Can you work these out from the model? Positions are in its coordinate system, mm. A direction names the side the tool comes from. Give positions to 0.01 mm unless a question says otherwise; leave off trailing zeros. Order: outer loops, then holes, each group sorted by start corner. A loop starts at its lowest first (then second) coordinate and runs counter-clockwise, first axis right, second up. Notation, with made-up numbers: M -39.5,50.25 L -24.5,50.25 A20 cw -24.5,80.25 Z; hole C 46.5,16 d1. An arc over 180 degrees is marked long. Use one line per item in the form item = value. Start each with the question number.
1. I need wall thicknesses on L1, parallel to X at y = 34.5, z = 57; L2, parallel to X at y = 75.5, z = 4.5; L3, parallel to Z at x = 164, y = 23. Which ranges of each line are inside material? Lowest first, please.
2. Will these pins go through, and if not, where does the flat tip stop? P1, Ø2, axis at y = 56, z = 12, coming from the +X side; P2, Ø8, axis at x = 34, z = 22.5, coming from the -Y side; P3, Ø1.6, axis at y = 83, z = 2, coming from the +X side; P4, Ø6, axis at x = -20.26, y = 0, coming from the +Z side.
3. I want a section at C-C, the plane z = 12. List the corners of the cut face in (x, y) for me, and give its area (3 significant figures).
4. I want a section at A-A, the plane x = 8.5. List the corners of the cut face in (y, z) for me, and give its area (3 significant figures).
5. For faces 4 (the face through (71.21, 54.46, 37.16)), 5 (the face through (71.14, -21.95, 19.46)), 6 (the face through (0, 82, 3)), 7 (the face through (142.16, 30.54, 65.24)), 8 (the face through (143.2, -15.65, 23.61)), which set-ups out of +Z, -Z, +X, -X, +Y, -Y let a thin tool reach every point of the face, with its end or its side?
6. We'd pull the mould along X, two halves only. Please class faces 1 (the face through (175.739, 24, 3)), 2 (the face through (-2.65, 32.53, 66.63)), 3 (the face through (72, -21, 7)): +X half, -X half, draft (parallel to the pull), parting line (faces both ways), or undercut.
```python
from build123d import *

# Parameters (mm, degrees)
F0_R          = 3.25
F0_W          = 147
F0_H          = 74
F0_W_2        = 5
F0_H_2        = 3
F1_DEPTH      = 7
F4_DEPTH      = 150.739
F4_DEPTH_BACK = 6.261
F5_W          = 147
F5_H          = 67.7437671193
F6_DEPTH      = 156.2
F7_R          = 1
F9_DEPTH      = 15
F10_R         = 1.75
F11_DEPTH     = 15


# Not quite as in the source:
# - a feature names something its author has since deleted; it is built from what else it names


with BuildPart() as f1:
    # F0 (on Top) → F1 (new body)
    with BuildSketch(Plane.XY):
        Polygon((30.7393903136, 82), (-31.2606096864, 82), (-31.2606096864, -32), (175.7393903136, -32), (175.7393903136, 82), (113.7393903136, 82), (108.7393903136, 82), (35.7393903136, 82), align=None)
        with Locations((-20.2606096864, 0)):
            Circle(F0_R, mode=Mode.SUBTRACT)
        with Locations((164.7393903136, 0)):
            Circle(F0_R, mode=Mode.SUBTRACT)
        with Locations((72.2393903136, 30)):
            Rectangle(F0_W, F0_H, mode=Mode.SUBTRACT)
        with Locations((33.2393903136, 83.5)):
            Rectangle(F0_W_2, F0_H_2)
        with Locations((111.2393903136, 83.5)):
            Rectangle(F0_W_2, F0_H_2)
    extrude(amount=F1_DEPTH)

    # F3 (on Right) → F4 (join, two sides)
    with BuildSketch(Plane.YZ) as f4_sk:
        Polygon((-13.2231451571, 7), (81.6844701767, 7), (33.2535275188, 76.1665542214), (-30.4304382476, 31.5745613287), align=None)
    extrude(amount=F4_DEPTH)
    extrude(f4_sk.sketch, amount=-F4_DEPTH_BACK)

    # F5 (on face) → F6 (cut)
    with BuildSketch(Plane(origin=(0, -24.8464988409, 35.4844777942), x_dir=(1, 0, 0), z_dir=(0, -0.5735764364, 0.8191520443))):
        with Locations((72.239, 32.0551522267)):
            Rectangle(F5_W, F5_H)
    extrude(amount=-F6_DEPTH, mode=Mode.SUBTRACT)

    # F7
    f7_edges = [f1.edges().sort_by_distance(p)[0] for p in [
        (111.23939, 85, 7),
        (33.23939, 85, 7),
        (35.73939, 85, 3.5),
        (30.73939, 85, 3.5),
        (108.73939, 85, 3.5),
        (113.73939, 85, 3.5),
    ]]
    fillet(f7_edges, radius=F7_R)

    # F8 (on face) → F9 (join)
    with BuildSketch(Plane(origin=(0, -24.8464988409, 35.4844777942), x_dir=(1, 0, 0), z_dir=(0, -0.5735764364, 0.8191520443))):
        with BuildLine():
            Line((-1.261, 65.9270357864), (3.739, 65.9270357864))
            ThreePointArc((3.739, 65.9270357864), (2.2745339059, 69.4625696923), (-1.261, 70.9270357864))
            Line((-1.261, 70.9270357864), (-6.261, 70.9270357864))
            Line((-6.261, 70.9270357864), (-6.261, 65.9270357864))
            ThreePointArc((-6.261, 65.9270357864), (-4.7965339059, 62.3915018804), (-1.261, 60.9270357864))
            Line((-1.261, 60.9270357864), (-1.261, 65.9270357864))
        make_face()
        with BuildLine():
            ThreePointArc((-1.261, 60.9270357864), (2.2745339059, 62.3915018804), (3.739, 65.9270357864))
            Line((3.739, 65.9270357864), (-1.261, 65.9270357864))
            Line((-1.261, 65.9270357864), (-1.261, 60.9270357864))
        make_face()
        with BuildLine():
            Line((145.739, -1.8167313329), (145.739, 3.1832686671))
            ThreePointArc((145.739, 3.1832686671), (142.2034660941, 1.718802573), (140.739, -1.8167313329))
            Line((140.739, -1.8167313329), (145.739, -1.8167313329))
        make_face()
        with BuildLine():
            ThreePointArc((140.739, 65.9270357864), (142.2034660941, 62.3915018804), (145.739, 60.9270357864))
            Line((145.739, 60.9270357864), (145.739, 65.9270357864))
            Line((145.739, 65.9270357864), (140.739, 65.9270357864))
        make_face()
        with BuildLine():
            Line((150.739, -6.8167313329), (150.739, -1.8167313329))
            ThreePointArc((150.739, -1.8167313329), (149.2745339059, 1.718802573), (145.739, 3.1832686671))
            Line((145.739, 3.1832686671), (145.739, -1.8167313329))
            Line((145.739, -1.8167313329), (140.739, -1.8167313329))
            ThreePointArc((140.739, -1.8167313329), (142.2034660941, -5.3522652388), (145.739, -6.8167313329))
            Line((145.739, -6.8167313329), (150.739, -6.8167313329))
        make_face()
        with BuildLine():
            ThreePointArc((145.739, 60.9270357864), (149.2745339059, 62.3915018804), (150.739, 65.9270357864))
            Line((150.739, 65.9270357864), (150.739, 70.9270357864))
            Line((150.739, 70.9270357864), (145.739, 70.9270357864))
            ThreePointArc((145.739, 70.9270357864), (142.2034660941, 69.4625696923), (140.739, 65.9270357864))
            Line((140.739, 65.9270357864), (145.739, 65.9270357864))
            Line((145.739, 65.9270357864), (145.739, 60.9270357864))
        make_face()
        with BuildLine():
            Line((-1.261, -1.8167313329), (3.739, -1.8167313329))
            ThreePointArc((3.739, -1.8167313329), (2.2745339059, 1.718802573), (-1.261, 3.1832686671))
            Line((-1.261, 3.1832686671), (-1.261, -1.8167313329))
        make_face()
    extrude(amount=-F9_DEPTH)

    # F10 (on face) → F11 (cut)
    with BuildSketch(Plane(origin=(0, -24.8464988409, 35.4844777942), x_dir=(1, 0, 0), z_dir=(0, -0.5735764364, 0.8191520443))):
        with Locations((145.739, -1.8167313329)):
            Circle(F10_R)
        with Locations((145.739, 65.9270357864)):
            Circle(F10_R)
        with Locations((-1.261, 65.9270357864)):
            Circle(F10_R)
        with Locations((-1.261, -1.8167313329)):
            Circle(F10_R)
    extrude(amount=-F11_DEPTH, mode=Mode.SUBTRACT)


solid = f1.part
```
Check result:
q1.L1 = -6.26 to -1.26, 145.74 to 150.74
q1.L2 = -31.26 to -1.26, 145.74 to 175.74
q1.L3 = 0 to 7
q2.P1 = 150.74
q2.P2 = -26.88
q2.P3 = 113.74
q2.P4 = through
q3.outline = M -6.26,-16.72 L 150.74,-16.72 L 150.74,78.18 L -6.26,78.18 Z; hole M -1.26,-10.62 L 145.74,-10.62 L 145.74,72.08 L -1.26,72.08 Z
q3.area = 2,740 mm2
q4.outline = M -32,0 L -7,0 L -7,6.83 L -26.33,34.44 L -30.43,31.57 L -13.22,7 L -32,7 Z; M 29.16,73.3 L 80.48,0 L 82,0 L 82,7 L 81.68,7 L 33.25,76.17 Z
q4.area = 775 mm2
q5.face_4 = -Z
q5.face_5 = +X, -X, -Y
q5.face_6 = +Z, -Z, -X, +Y
q5.face_7 = -Z, -Y
q5.face_8 = none
q6.face_1 = +X half
q6.face_2 = undercut
q6.face_3 = draft
